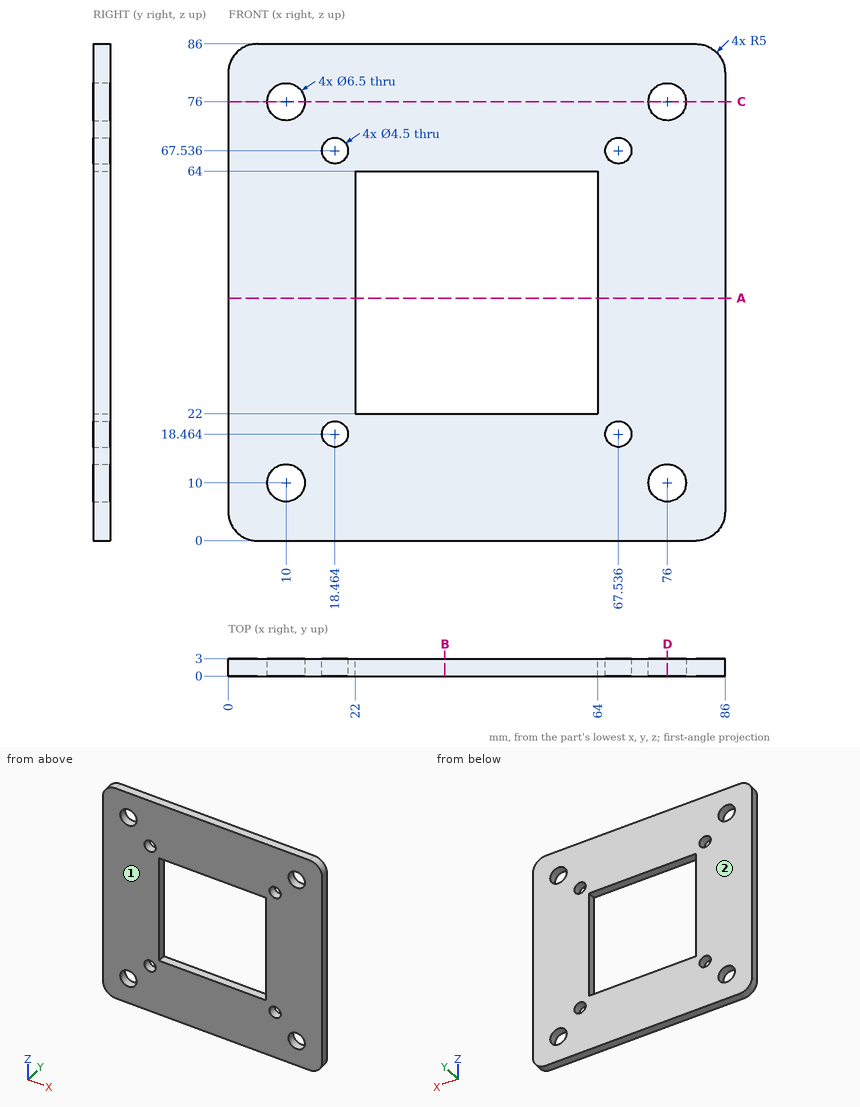
Job drawing, mm, ordinate dimensions from the low corner. One solid piece. Round coordinates to 2 decimals unless told otherwise and drop trailing zeros. Write each loop counter-clockwise with the first axis right and the second up, starting at its lowest first coordinate (ties: lowest second). Pieces come first, ordered by that corner, then holes. Notation, with made-up numbers: (28.25, 67) -> (36.25, 67) arc R14 cw to (36.25, 91) -> close; hole circle Ø11 at (0, -22). An arc over 180 degrees is marked (long way). Answer as CSV lines item,"result".
1. Slice it at C-C, the plane z = 76. List the corners of the cut face in (x, y).
Resolved:
outline,"(0, 0) -> (6.75, 0) -> (6.75, 3) -> (0, 3) -> close; (13.25, 0) -> (72.75, 0) -> (72.75, 3) -> (13.25, 3) -> close; (79.25, 0) -> (86, 0) -> (86, 3) -> (79.25, 3) -> close"
2. Slice it at B-B, the plane x = 37.5. List the corners of the cut face in (y, z).
Resolved:
outline,"(0, 0) -> (3, 0) -> (3, 22) -> (0, 22) -> close; (0, 64) -> (3, 64) -> (3, 86) -> (0, 86) -> close"
3. Slice it at D-D, the plane x = 76. List the corners of the cut face in (y, z), plus the area to 3 significant figures.
Resolved:
outline,"(0, 0) -> (3, 0) -> (3, 6.75) -> (0, 6.75) -> close; (0, 13.25) -> (3, 13.25) -> (3, 72.75) -> (0, 72.75) -> close; (0, 79.25) -> (3, 79.25) -> (3, 86) -> (0, 86) -> close"
area,"219 mm²"
4. Mould opens along Y. For the marked faces 1 and 2 say: +Y half, -Y half, draft (parallel to the pull), parting line (faces both ways), or undercut.
Resolved:
face 1,"-Y half"
face 2,"+Y half"
5. Drill centre lines: line 1 (Z direction, x = 10, y = 2.1); line 2 (X direction, y = 2.8, z = 67.5) (1 decimal); line 3 (X direction, y = 0.75, z = 43). Where is each one in solid material? Low to high.
Resolved:
line 1,"0 to 6.75, 13.25 to 72.75, 79.25 to 86"
line 2,"0 to 16.2, 20.7 to 65.3, 69.8 to 86"
line 3,"0 to 22, 64 to 86"
6. Slice it at A-A, the plane z = 42. List the corners of the cut face in (x, y).
Resolved:
outline,"(0, 0) -> (22, 0) -> (22, 3) -> (0, 3) -> close; (64, 0) -> (86, 0) -> (86, 3) -> (64, 3) -> close"
